Model file for the job. Use its own axes, mm. Round coordinates to 2 decimals unless told otherwise and drop trailing zeros. Loops run counter-clockwise (first coordinate to the right, second up) from the corner with the lowest first, then second, coordinate; pieces in that order, holes last. Notation, with made-up numbers: M 76.25,-39 L 117.25,-39 A22 cw 117.25,-7 Z; hole C -11.5,-8 d4. An arc over 180 degrees is marked long. Answer in a Markdown table with one row per item.
from build123d import *

# Parameters (mm, degrees)
ESQUISSE1_R        = 1.5
BOSS_EXTRU_1_DEPTH = 5


with BuildPart() as part:
    # Esquisse1 → Boss.-Extru.1 (new body)
    with BuildSketch(Plane.XY):
        with BuildLine():
            Line((0, 8), (17.728942549, 8))
            ThreePointArc((17.728942549, 8), (38.177418085, 0.047486569), (59.342105263, 5.830101749))
            ThreePointArc((59.342105263, 5.830101749), (63.350754016, 5.193679781), (63.05640037, 1.145513075))
            ThreePointArc((63.05640037, 1.145513075), (52.401995882, -5.630136101), (40, -8))
            Line((40, -8), (0, -8))
            Line((0, -8), (-15, -8))
            ThreePointArc((-15, -8), (-23, 0), (-15, 8))
            Line((-15, 8), (0, 8))
        make_face()
        Circle(ESQUISSE1_R, mode=Mode.SUBTRACT)
        with Locations((-15, 0)):
            Circle(ESQUISSE1_R, mode=Mode.SUBTRACT)
    extrude(amount=BOSS_EXTRU_1_DEPTH)


solid = part.part
1. Saw through at B-B (y = 5). Write the cut outline in (x, z) (3 decimals), and give its area (3 significant figures).
Verdict:
| item | result |
|---|---|
| outline | M -21.245,0 L 21.972,0 L 21.972,5 L -21.245,5 Z; M 58.028,0 L 63.492,0 L 63.492,5 L 58.028,5 Z |
| area | 243 mm² |
2. Saw through at D-D (y = -3.5). Write the cut outline in (x, z), and give its area (3 significant figures).
Verdict:
| item | result |
|---|---|
| outline | M -22.19,0 L 56.81,0 L 56.81,5 L -22.19,5 Z |
| area | 395 mm² |
3. Mould opens along X. For faces 1 (the flat face through (11, 0, 5)), 2 (the cylindrical face through (52.567, -5.564, 2.465)), 3 (the cylindrical face through (37.865, 0.065, 2.465)), 4 (the cylindrical face through (-23, 0, 2)) say: +X half, -X half, draft (parallel to the pull), parting line (faces both ways), or undercut.
Verdict:
| item | result |
|---|---|
| face 1 | draft |
| face 2 | +X half |
| face 3 | undercut |
| face 4 | -X half |
4. Pin check, flat tips, straight feed: pin 1 (4 mm diameter, centred on x = 1.5, y = -0.5, fed in from -Z); pin 2 (1 mm diameter, centred on x = 28.5, z = 1, fed in from +Y); pin 3 (3 mm diameter, centred on y = -1, z = 3, fed in from +X); pin 4 (1 mm diameter, centred on y = 3.5, z = 4, fed in from -X). Stop position of each tip, or through.
Verdict:
| item | result |
|---|---|
| pin 1 | stops at z = 0 |
| pin 2 | stops at y = 2.12 |
| pin 3 | stops at x = 62.35 |
| pin 4 | stops at x = -22.42 |
5. Saw through at A-A (x = 0). Write the cut outline in (y, z), and give its area (3 significant figures).
Verdict:
| item | result |
|---|---|
| outline | M -8,0 L -1.5,0 L -1.5,5 L -8,5 Z; M 1.5,0 L 8,0 L 8,5 L 1.5,5 Z |
| area | 65.0 mm² |
6. Saw through at C-C (z = 2.8). Write the cut outline in (x, y).
Verdict:
| item | result |
|---|---|
| outline | M -15,-8 L 40,-8 A33.64 ccw 63.06,1.15 A3 ccw 59.34,5.83 A35 cw 17.73,8 L -15,8 A8 ccw Z; hole C -15,0 d3; hole C 0,0 d3 |
7. Wall check: probe 1 along Y at (x, z) = (-15, 1.9); probe 2 along X at (y, z) = (4.75, 2.5); probe 3 along Y at (x, z) = (-0.5, 3.05). Give the ranges that are in metal, low to high.
Verdict:
| item | result |
|---|---|
| probe 1 | y = -8 to -1.5, 1.5 to 8 |
| probe 2 | x = -21.44 to 22.39, 57.61 to 63.64 |
| probe 3 | y = -8 to -1.41, 1.41 to 8 |
